Verification items for this drawing (mm, ordinates from the low corner). Coordinates: 2 decimals unless noted, no trailing zeros. Loops run counter-clockwise (first coordinate to the right, second up) from the corner with the lowest first, then second, coordinate; pieces in that order, holes last. Notation, with made-up numbers: (59.25, 17.25) -> (71.25, 17.25) arc R20 cw to (71.25, 44.25) -> close; hole circle Ø10 at (77.5, -8). An arc over 180 degrees is marked (long way). Write item = value, one per line.
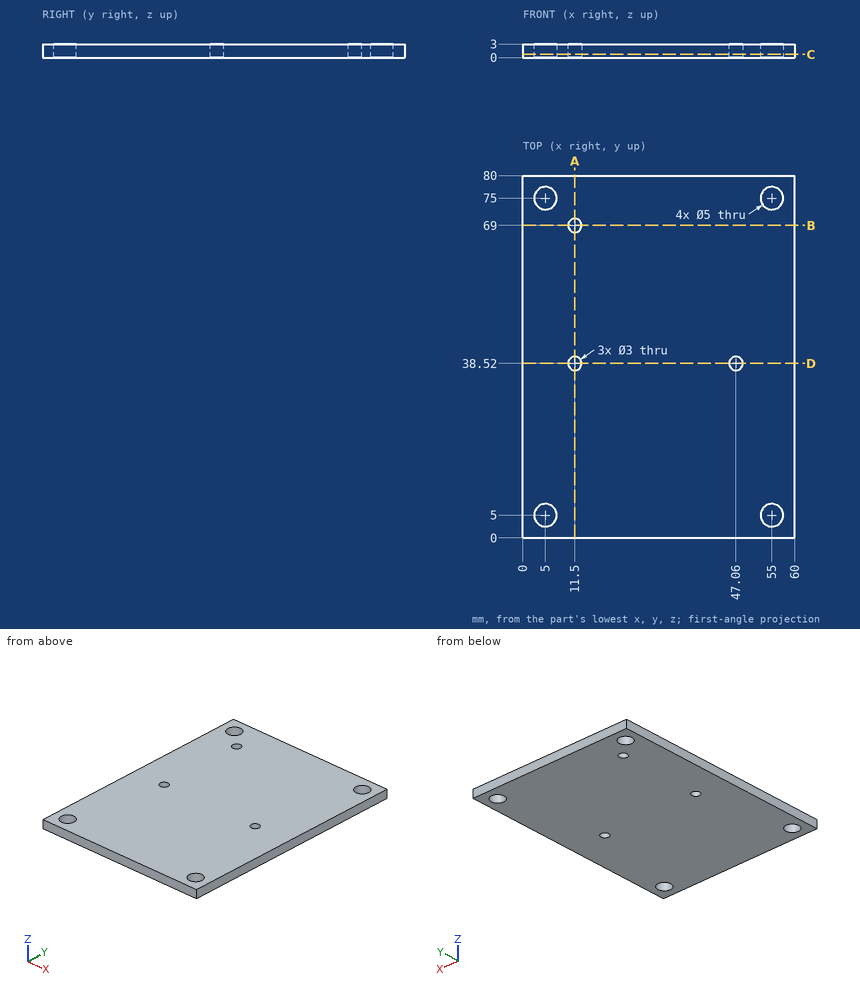
1) Sectioned sample at B-B, the plane y = 69. Record the cut outline in (x, z), plus the area to 3 significant figures.
Ans:
outline = (0, 0) -> (10, 0) -> (10, 3) -> (0, 3) -> close; (13, 0) -> (60, 0) -> (60, 3) -> (13, 3) -> close
area = 171 mm2
2) Sectioned sample at A-A, the plane x = 11.5. Record the cut outline in (y, z).
Ans:
outline = (0, 0) -> (37.02, 0) -> (37.02, 3) -> (0, 3) -> close; (40.02, 0) -> (67.5, 0) -> (67.5, 3) -> (40.02, 3) -> close; (70.5, 0) -> (80, 0) -> (80, 3) -> (70.5, 3) -> close
3) Sectioned sample at C-C, the plane z = 0.7. Record the cut outline in (x, y), plus the area to 3 significant figures.
Ans:
outline = (0, 0) -> (60, 0) -> (60, 80) -> (0, 80) -> close; hole circle Ø5 at (5, 5); hole circle Ø5 at (5, 75); hole circle Ø3 at (11.5, 38.52); hole circle Ø3 at (11.5, 69); hole circle Ø3 at (47.06, 38.52); hole circle Ø5 at (55, 5); hole circle Ø5 at (55, 75)
area = 4,700 mm2
4) Material ranges on line 1 (Y direction, x = 11.5, z = 2.35); line 2 (X direction, y = 75, z = 0.8); line 3 (Y direction, x = 55, z = 2.1), recorded low to high.
Ans:
line_1 = 0 to 37.02, 40.02 to 67.5, 70.5 to 80
line_2 = 0 to 2.5, 7.5 to 52.5, 57.5 to 60
line_3 = 0 to 2.5, 7.5 to 72.5, 77.5 to 80
5) Sectioned sample at D-D, the plane y = 38.52. Record the cut outline in (x, z).
Ans:
outline = (0, 0) -> (10, 0) -> (10, 3) -> (0, 3) -> close; (13, 0) -> (45.56, 0) -> (45.56, 3) -> (13, 3) -> close; (48.56, 0) -> (60, 0) -> (60, 3) -> (48.56, 3) -> close
